Check sheet for the drawn part. Datum: minimum x, y, z corner. Units: mm. A direction names the side the tool comes from. Coordinates: 2 decimals unless noted, no trailing zeros. Order: outer loops, then holes, each group sorted by start corner. A loop starts at its lowest first (then second) coordinate and runs counter-clockwise, first axis right, second up.
1. Set-up check for the marked faces 4, 5, 6 and 7: record each of +Z, -Z, +X, -X, +Y, -Y from which the full face is reachable in a straight line by a thin tool's end or side.
2. Thickness scan on line 1 (X direction, y = 17.2, z = 45); line 2 (X direction, y = 16, z = 23.5); line 3 (Y direction, x = 26, z = 9.5). Record the ranges inside material, lowest first.
3. Cross-section at D-D (z = 13.5). Enter the section's corners in (x, y), then the cut area to 3 significant figures.
4. Draft check along X on the marked faces 1, 2 and 3. Enter one of: released by +X, released by -X, zero draft, split by the parting line, or undercut.
5. Gauge pin test, flat ends, axial feed: pin 1 Ø2 at (x, y) = (29, 18.5) entering from -Z; pin 2 Ø5 at (x, z) = (23.5, 24.5) entering from +Y; pin 3 Ø5 at (x, z) = (27, 37.5) entering from -Y. Record the tip position at first contact, or that the pin passes through.
6. Cross-section at B-B (x = 32). Enter the section's corners in (y, z), then the cut area to 3 significant figures.
7. Cross-section at A-A (z = 45). Enter the section's corners in (x, y).
8. Cross-section at C-C (x = 20). Enter the section's corners in (y, z).
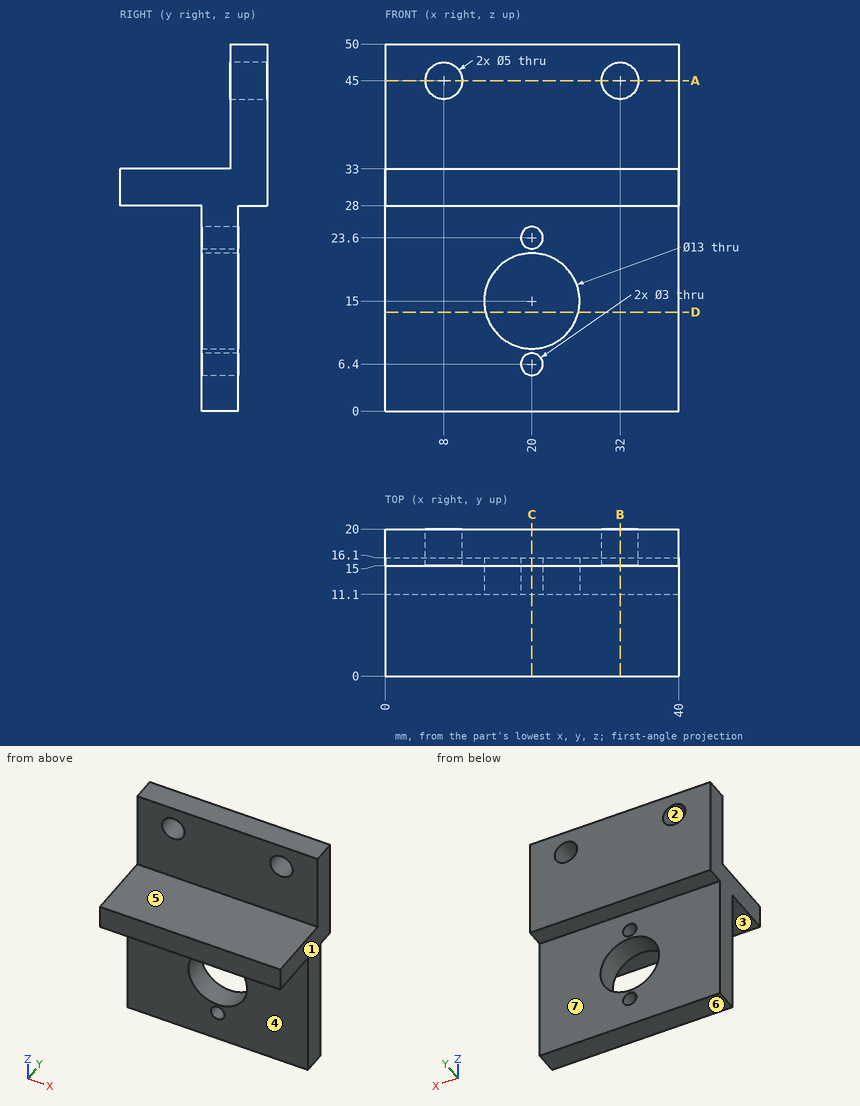
Data:
1. face 4: -Z, +X, -X, -Y
1. face 5: +Z, +X, -X, -Y
1. face 6: -Z, +X, -X, +Y, -Y
1. face 7: -Z, +X, -X, +Y
2. line 1: x = 0 to 5.5, 10.5 to 29.5, 34.5 to 40
2. line 2: x = 0 to 18.5, 21.5 to 40
2. line 3: y = 11.1 to 16.1
3. outline: (0, 11.1) - (13.68, 11.1) - (13.68, 16.1) - (0, 16.1) - close; (26.32, 11.1) - (40, 11.1) - (40, 16.1) - (26.32, 16.1) - close
3. area: 137 mm2
4. face 1: released by +X
4. face 2: undercut
4. face 3: zero draft
5. pin 1: stops at z = 28
5. pin 2: stops at y = 16.1
5. pin 3: stops at y = 15
6. outline: (0, 28) - (11.1, 28) - (11.1, 0) - (16.1, 0) - (16.1, 28) - (20, 28) - (20, 42.5) - (15, 42.5) - (15, 33) - (0, 33) - close; (15, 47.5) - (20, 47.5) - (20, 50) - (15, 50) - close
6. area: 300 mm2
7. outline: (0, 15) - (5.5, 15) - (5.5, 20) - (0, 20) - close; (10.5, 15) - (29.5, 15) - (29.5, 20) - (10.5, 20) - close; (34.5, 15) - (40, 15) - (40, 20) - (34.5, 20) - close
8. outline: (0, 28) - (11.1, 28) - (11.1, 25.1) - (16.1, 25.1) - (16.1, 28) - (20, 28) - (20, 50) - (15, 50) - (15, 33) - (0, 33) - close; (11.1, 0) - (16.1, 0) - (16.1, 4.9) - (11.1, 4.9) - close; (11.1, 7.9) - (16.1, 7.9) - (16.1, 8.5) - (11.1, 8.5) - close; (11.1, 21.5) - (16.1, 21.5) - (16.1, 22.1) - (11.1, 22.1) - close
